```python
from build123d import *

# Parameters (mm, degrees)
SKETCH1_W            = 100
SKETCH1_H            = 73.5
SKETCH1_W_2          = 93
SKETCH1_H_2          = 66.5
BOSS_EXTRUDE1_DEPTH  = 10
SKETCH2_W            = 100
SKETCH2_H            = 73.5
BOSS_EXTRUDE2_DEPTH  = 3
SKETCH3_R            = 3.5
BOSS_EXTRUDE8_DEPTH  = 3.5
SKETCH4_W            = 12
SKETCH4_H            = 15
CUT_EXTRUDE4_DEPTH   = 3
SKETCH7_W            = 100
SKETCH7_H            = 3
BOSS_EXTRUDE12_DEPTH = 12
SKETCH8_W            = 21
SKETCH8_H            = 3
SKETCH8_W_2          = 10.5
CUT_EXTRUDE2_DEPTH   = 12
BOSS_EXTRUDE13_DEPTH = 29.5
BOSS_EXTRUDE14_DEPTH = 29.5
CUT_EXTRUDE3_DEPTH   = 93.5
BOSS_EXTRUDE15_DEPTH = 93


with BuildPart() as part:
    # Sketch1 → Boss-Extrude1 (new body)
    with BuildSketch(Plane.XY):
        Rectangle(SKETCH1_W, SKETCH1_H)
        Rectangle(SKETCH1_W_2, SKETCH1_H_2, mode=Mode.SUBTRACT)
    extrude(amount=BOSS_EXTRUDE1_DEPTH)

    # Sketch2 → Boss-Extrude2 (add)
    with BuildSketch(Plane(origin=(0, 0, 0), x_dir=(-1, 0, 0), z_dir=(0, 0, -1))):
        Rectangle(SKETCH2_W, SKETCH2_H)
    extrude(amount=BOSS_EXTRUDE2_DEPTH)

    # Sketch3 → Boss-Extrude8 (add)
    with BuildSketch(Plane(origin=(50, 0, 0), x_dir=(0, 0, -1), z_dir=(1, 0, 0))):
        with BuildLine():
            Line((-10, -21.75), (-18, -21.75))
            ThreePointArc((-18, -21.75), (-25.303809073, -27.545777883), (-21.319283456, -35.975500527))
            Line((-21.319283456, -35.975500527), (-18, -36.75))
            Line((-18, -36.75), (-10, -36.75))
            Line((-10, -36.75), (-10, -21.75))
        make_face()
        with Locations(Location((-18, -29.25, 0), (0, 0, 90))):
            Circle(SKETCH3_R, mode=Mode.SUBTRACT)
    extrude(amount=-BOSS_EXTRUDE8_DEPTH)

    # Sketch4 → Cut-Extrude4 (cut)
    with BuildSketch(Plane.ZY.offset(50)):
        with Locations((4, -29.25)):
            Rectangle(SKETCH4_W, SKETCH4_H)
    extrude(amount=-CUT_EXTRUDE4_DEPTH, mode=Mode.SUBTRACT)

    # Sketch7 → Boss-Extrude12 (add)
    with BuildSketch(Plane.XY.offset(10)):
        with Locations((0, 35.25)):
            Rectangle(SKETCH7_W, SKETCH7_H)
    extrude(amount=BOSS_EXTRUDE12_DEPTH)

    # Sketch8 → Cut-Extrude2 (cut)
    with BuildSketch(Plane.XY.offset(22)):
        with Locations((0, 35.25)):
            Rectangle(SKETCH8_W, SKETCH8_H)
        with Locations((-44.75, 35.25)):
            Rectangle(SKETCH8_W_2, SKETCH8_H)
        with Locations((44.75, 35.25)):
            Rectangle(SKETCH8_W_2, SKETCH8_H)
    extrude(amount=-CUT_EXTRUDE2_DEPTH, mode=Mode.SUBTRACT)

    # Sketch9 → Boss-Extrude13 (add)
    with BuildSketch(Plane(origin=(39.5, 0, 0), x_dir=(0, 0, -1), z_dir=(1, 0, 0))):
        Polygon((-22, 33.75), (-20.75, 32.5), (-17.75, 32.5), (-16.5, 33.75), align=None)
    extrude(amount=-BOSS_EXTRUDE13_DEPTH)

    # Sketch10 → Boss-Extrude14 (add)
    with BuildSketch(Plane(origin=(-10.5, 0, 0), x_dir=(0, 0, -1), z_dir=(1, 0, 0))):
        Polygon((-22, 33.75), (-20.75, 32.5), (-17.75, 32.5), (-16.5, 33.75), align=None)
    extrude(amount=-BOSS_EXTRUDE14_DEPTH)

    # Sketch11 → Cut-Extrude3 (cut)
    with BuildSketch(Plane(origin=(39.5, 0, 0), x_dir=(0, 0, -1), z_dir=(1, 0, 0))):
        Polygon((-19.25, 36.75), (-19.25, 35.75), (-18.25, 36.75), align=None)
        Polygon((-19.25, 36.75), (-20.25, 36.75), (-19.25, 35.75), align=None)
        Polygon((-21.133974596, 35.25), (-22, 36.75), (-22, 35.25), align=None)
        Polygon((-22, 33.75), (-21.133974596, 35.25), (-22, 35.25), align=None)
    extrude(amount=-CUT_EXTRUDE3_DEPTH, mode=Mode.SUBTRACT)

    # Sketch12 → Boss-Extrude15 (add)
    with BuildSketch(Plane.ZY.offset(-46.5)):
        Polygon((10, -36.75), (13.5, -36.75), (10, -33.25), align=None)
    extrude(amount=BOSS_EXTRUDE15_DEPTH)


solid = part.part
```
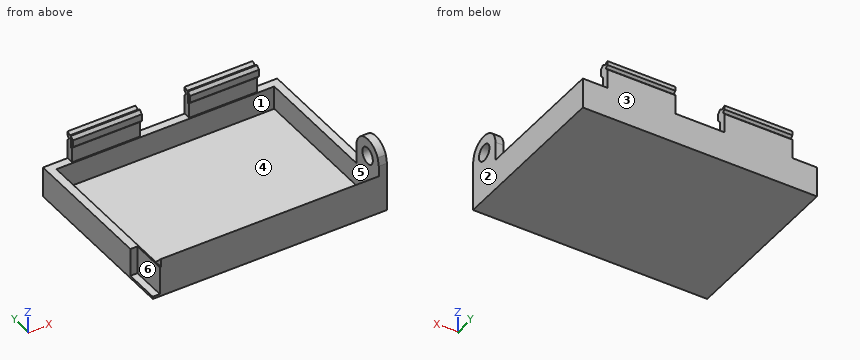
Could you check a few things on this model? Use its own coordinates, in mm. Face numbers are marked on the shaded views. A direction names the side the tool comes from. Give positions to 0.01 mm unless a question says otherwise; leave off trailing zeros. Write each loop counter-clockwise with the first axis right and the second up, starting at its lowest first coordinate (ties: lowest second). Pieces come first, ordered by that corner, then holes. Notation, with made-up numbers: (82, 70.25) - (88, 70.25) arc R23 cw to (88, 105.25) - close; hole circle Ø6 at (43.25, 6.25). An arc over 180 degrees is marked (long way). One line per item, written item: value. Start each with the question number.
Item 1: Imagine slicing it at D-D, the plane y = -18.5. List the corners of the cut face in (x, z) for me.
Item 2: Please list where these lines run through material, in increasing order: line 1 (Z direction, x = 48, y = -29); line 2 (Y direction, x = -7, z = 2.5); line 3 (X direction, y = 8, z = 0.75). Write a range as from..to.
Item 3: Imagine slicing it at A-A, the plane y = -29.25. List the corners of the cut face in (x, z) for me, and give its area (3 significant figures).
Item 4: If we mould it in two halves opening along Y, with no side actions, what happens to the marked faces 3, 4, 5 and 6? For each: +Y half, -Y half, draft (parallel to the pull), parting line (faces both ways), or undercut.
Item 5: Which directions (+Z, -Z, +X, -X, +Y, -Y) give clear straight access to the entire face, cutting with the end or side of a thin tool? Please do the marked faces 1 and 2.
Item 6: Imagine slicing it at C-C, the plane z = 5.75. List the corners of the cut face in (x, y) for me, and give its area (3 significant figures).
Item 7: Imagine slicing it at B-B, the plane x = 27. List the corners of the cut face in (y, z) for me.
Item 8: I'm going to push flat-ended pins straight in: pin 1 (2.5 mm diameter, centred on x = -49, y = -32, fed in from +Z); pin 2 (1.5 mm diameter, centred on y = 35.5, z = 17, fed in from -X); pin 3 (3.5 mm diameter, centred on x = -23, z = 19.5, fed in from -Y); pin 4 (4 mm diameter, centred on y = -5, z = 12.5, fed in from -X). Where does each tip first touch, or does it pass through?
Geometry says:
1. outline: (-50, -3) - (50, -3) - (50, 10) - (46.5, 10) - (46.5, 0) - (-46.5, 0) - (-46.5, 10) - (-50, 10) - close
2. line 1: -3..14.51, 21.49..25.5
2. line 2: -36.75..-33.25, 33.25..36.75
2. line 3: -50..-46.5, 46.5..50
3. outline: (-50, -3) - (50, -3) - (50, 14.5) - (46.5, 14.5) - (46.5, 0) - (-46.5, 0) - (-46.5, 10) - (-47, 10) - (-47, -2) - (-50, -2) - close; (46.5, 21.5) - (50, 21.5) - (50, 25.5) - (46.5, 25.5) - close
3. area: 364 mm^2
4. face 3: +Y half
4. face 4: undercut
4. face 5: undercut
4. face 6: draft
5. face 1: none
5. face 2: +Z, -Z, +X, +Y, -Y
6. outline: (-50, -21.75) - (-47, -21.75) - (-47, -36.75) - (50, -36.75) - (50, 36.75) - (-50, 36.75) - close; hole (-46.5, -33.25) - (46.5, -33.25) - (46.5, 33.25) - (-46.5, 33.25) - close
6. area: 1,120 mm^2
7. outline: (-36.75, -3) - (36.75, -3) - (36.75, 18.25) - (35.75, 19.25) - (36.75, 20.25) - (36.75, 22) - (35.25, 21.13) - (33.75, 22) - (32.5, 20.75) - (32.5, 17.75) - (33.75, 16.5) - (33.75, 10) - (33.25, 10) - (33.25, 0) - (-33.25, 0) - (-33.25, 10) - (-36.75, 13.5) - close
8. pin 1: z = -2
8. pin 2: x = -39.5
8. pin 3: y = 32.5
8. pin 4: through
